from build123d import *

# Parameters (mm, degrees)
F1_DEPTH        = 25
F2_DEPTH        = 50
F2_COPIES_COUNT = 4
F4_DEPTH        = 25.001
F4_COPIES_COUNT = 4


# Not quite as in the source:
# - a pattern or mirror of a feature is missing from the dataset's text; its kind, count and spacing are read off the source's solid


with BuildPart() as f1:
    # F0 (on Top) → F1 (new body)
    with BuildSketch(Plane.XY):
        with BuildLine():
            ThreePointArc((-7.4765908914, 46.9078947368), (-30.8310876605, -36.1343885194), (47.5, 0))
            ThreePointArc((47.5, 0), (36.1343885194, 30.8310876605), (7.4765908914, 46.9078947368))
            ThreePointArc((7.4765908914, 46.9078947368), (0, 40), (-7.4765908914, 46.9078947368))
        make_face()
        with BuildLine():
            ThreePointArc((-7.4765908914, 46.9078947368), (0, 40), (7.4765908914, 46.9078947368))
            ThreePointArc((7.4765908914, 46.9078947368), (0, 47.5), (-7.4765908914, 46.9078947368))
        make_face()
    extrude(amount=F1_DEPTH)

    # F0 (on Top) → F2 (join)
    with BuildSketch(Plane.XY):
        with BuildLine():
            ThreePointArc((-7.4765908914, 46.9078947368), (0, 40), (7.4765908914, 46.9078947368))
            ThreePointArc((7.4765908914, 46.9078947368), (0, 47.5), (-7.4765908914, 46.9078947368))
        make_face()
        with BuildLine():
            ThreePointArc((-7.4765908914, 46.9078947368), (0, 47.5), (7.4765908914, 46.9078947368))
            ThreePointArc((7.4765908914, 46.9078947368), (7.4941454378, 47.2037160867), (7.5, 47.5))
            ThreePointArc((7.5, 47.5), (-0.2962839133, 54.9941454378), (-7.4765908914, 46.9078947368))
        make_face()
    f2 = extrude(amount=F2_DEPTH)

    # F2_copies: F2 ×4 about axis
    f2_copies_axis = Axis((0, 0, 0), (0, 0, 1))
    for i in range(1, F2_COPIES_COUNT):
        add(f2.rotate(f2_copies_axis, i * 360 / F2_COPIES_COUNT))

    # F3 (on face) → F4 (cut, through all)
    with BuildSketch(Plane.XY.offset(25)):
        with BuildLine():
            ThreePointArc((42.3863974889, 21.4392935498), (33.5875721064, 33.5875721064), (21.4392935498, 42.3863974889))
            ThreePointArc((21.4392935498, 42.3863974889), (22.9809703886, 22.9809703886), (42.3863974889, 21.4392935498))
        make_face()
    f4 = extrude(amount=-F4_DEPTH, mode=Mode.SUBTRACT)

    # F4_copies: F4 ×4 about axis
    f4_copies_axis = Axis((0, 0, 0), (0, 0, 1))
    for i in range(1, F4_COPIES_COUNT):
        add(f4.rotate(f4_copies_axis, i * 360 / F4_COPIES_COUNT), mode=Mode.SUBTRACT)


solid = f1.part
The listing builds one solid part. Answer for the finished solid, in the listing's coordinates (mm). A direction names the side the tool comes from. Coordinates: 2 decimals unless noted, no trailing zeros. Write each loop counter-clockwise with the first axis right and the second up, starting at its lowest first coordinate (ties: lowest second). Pieces come first, ordered by that corner, then holes. Notation, with made-up numbers: M -14,-13 L 1,-13 A31 ccw 1,25 Z; hole C 31,-12 d10. An arc over 180 degrees is marked long. Put each result on its own line as item: value. Start each with the question number.
1. A cutting plane is placed at A-A on z = 28.5. Write down the section's boundary in (x, y), then the cut area to 3 significant figures.
2. A cutting plane is placed at D-D on z = 7. Write down the section's boundary in (x, y), then the cut area to 3 significant figures.
3. For a pull along X with two mould halves and no side action, classify faces 1 (the flat face through (-48, 0, 50)), 2 (the cylindrical face through (-45.16, 14.73, 12.32)), 3 (the cylindrical face through (23.193, -22.773, 12.675)) as pulls with the +X half, pulls with the -X half, needs draft (parallel to the pull), parting line crosses it, or undercut.
4. Consider line 1 (Z direction, x = -21.5, y = 2.5); line 2 (Y direction, x = 47, z = 44.5); line 3 (X direction, y = 47.5, z = 21). Determine where each line is inside the solid, lowest interval first. Write a range as from..to.
5. Flat-ended cylindrical pins translate along their axes: P1, Ø6, axis at x = -20.5, z = 15.5, coming from the +Y side; P2, Ø2, axis at y = 7.5, z = 15, coming from the -X side; P3, Ø1.5, axis at y = -38.5, z = 36.5, coming from the -X side; P4, Ø4, axis at y = -26, z = 5.5, coming from the -X side. Find the tip coordinate at first contact, or state that the pin passes through.
6. A cutting plane is placed at B-B on y = 0. Write down the section's boundary in (x, z), then the cut area to 3 significant figures.
7. Which of the six approach directions +Z, -Z, +X, -X, +Y, -Y give full straight-line access (tool end or side, diameter ignored) to faces 4 (the flat face through (-1, 1, 25)), 5 (the flat face through (0, -48, 50))?
Resolved:
1. outline: C -47.5,0 d15; C 0,-47.5 d15; C 0,47.5 d15; C 47.5,0 d15
1. area: 707 mm2
2. outline: M -46.91,-7.48 A47.5 ccw -42.39,-21.44 A15 cw -21.44,-42.39 A47.5 ccw -7.48,-46.91 A7.5 ccw long 7.48,-46.91 A47.5 ccw 21.44,-42.39 A15 cw 42.39,-21.44 A47.5 ccw 46.91,-7.48 A7.5 ccw long 46.91,7.48 A47.5 ccw 42.39,21.44 A15 cw 21.44,42.39 A47.5 ccw 7.48,46.91 A7.5 ccw long -7.48,46.91 A47.5 ccw -21.44,42.39 A15 cw -42.39,21.44 A47.5 ccw -46.91,7.48 A7.5 ccw long Z
2. area: 6,130 mm2
3. face 1: needs draft
3. face 2: pulls with the -X half
3. face 3: undercut
4. line 1: z = 0..25
4. line 2: y = -7.48..7.48
4. line 3: x = -7.5..7.5
5. P1: stops at y = 44.16
5. P2: stops at x = -51.24
5. P3: passes through
5. P4: stops at x = -22.05
6. outline: M -55,0 L 55,0 L 55,50 L 40,50 L 40,25 L -40,25 L -40,50 L -55,50 Z
6. area: 3,500 mm2
7. face 4: +Z
7. face 5: +Z, +X, -X, +Y, -Y
